Input: dimensioned drawing with shaded views. Units: mm. Origin: part minimum x, y, z. A direction names the side the tool comes from. Give positions to 0.01 mm unless a question says otherwise; leave off trailing zeros. Order: outer loops, then holes, each group sorted by start corner. A loop starts at its lowest first (then second) coordinate and runs counter-clockwise, first axis right, second up.
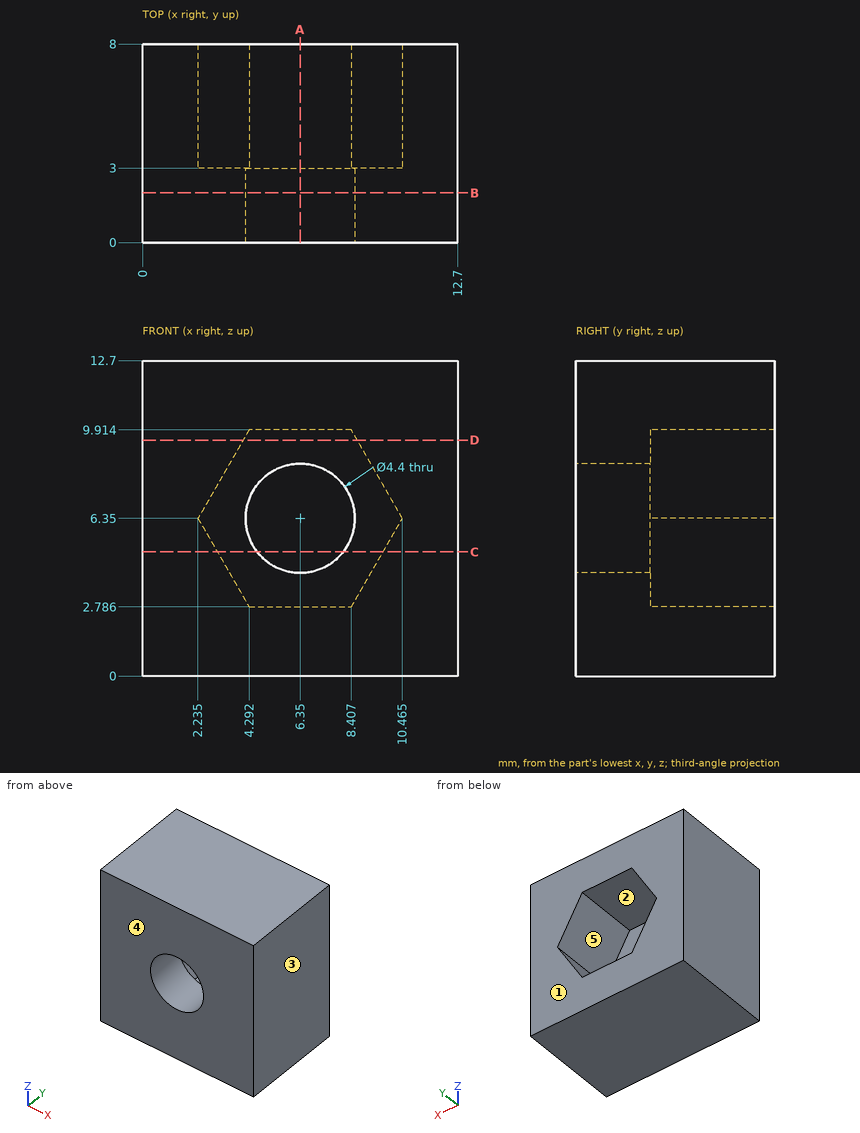
1) Pin query (flat end, axial travel): pin 1 (4 mm diameter, centred on x = 6.35, z = 6.35, fed in from +Y). Return the tip coordinate at first contact, or that it passes through.
Report:
pin 1: passes through
2) Material intervals for L1, parallel to Z at x = 5.5, y = 5.5; L2, parallel to Z at x = 6.35, y = 1.25, sorted ascending.
Report:
L1: z = 0 to 2.79, 9.91 to 12.7
L2: z = 0 to 4.15, 8.55 to 12.7
3) Draft query along X for the marked faces 3, 4 and 5. Return one class per face: +X half, -X half, draft (parallel to the pull), parting line (faces both ways), or undercut.
Report:
face 3: +X half
face 4: draft
face 5: undercut
4) Section query C-C, the plane z = 5. Return the cut outline in (x, y) (1 decimal).
Report:
outline: (0, 0) - (4.6, 0) - (4.6, 3) - (3, 3) - (3, 8) - (0, 8) - close; (8.1, 0) - (12.7, 0) - (12.7, 8) - (9.7, 8) - (9.7, 3) - (8.1, 3) - close
5) Section query B-B, the plane y = 2. Return the cut outline in (x, z).
Report:
outline: (0, 0) - (12.7, 0) - (12.7, 12.7) - (0, 12.7) - close; hole circle Ø4.4 at (6.35, 6.35)
6) Section query D-D, the plane z = 9.5. Return the cut outline in (x, y).
Report:
outline: (0, 0) - (12.7, 0) - (12.7, 8) - (8.65, 8) - (8.65, 3) - (4.05, 3) - (4.05, 8) - (0, 8) - close
7) Reachability of the marked faces 1 and 2 from +Z, -Z, +X, -X, +Y, -Y: full face, straight path, thin tool, end or side. Return the list, or none.
Report:
face 1: +Z, -Z, +X, -X, +Y
face 2: +Y
8) Section query A-A, the plane x = 6.35. Return the cut outline in (y, z).
Report:
outline: (0, 0) - (8, 0) - (8, 2.79) - (3, 2.79) - (3, 4.15) - (0, 4.15) - close; (0, 8.55) - (3, 8.55) - (3, 9.91) - (8, 9.91) - (8, 12.7) - (0, 12.7) - close
